```python
from build123d import *

# Parameters (mm, degrees)
SKETCH1_W           = 60
SKETCH1_H           = 400
BOSS_EXTRUDE1_DEPTH = 5
SKETCH2_R           = 30
BOSS_EXTRUDE2_DEPTH = 3
SKETCH3_R           = 3
BOSS_EXTRUDE3_DEPTH = 13
SKETCH4_R           = 4
BOSS_EXTRUDE4_DEPTH = 5
LPATTERN1_COUNT     = 8
LPATTERN1_PITCH     = 40


with BuildPart() as part:
    # Sketch1 → Boss-Extrude1 (new body)
    with BuildSketch(Plane.XY):
        Rectangle(SKETCH1_W, SKETCH1_H)
    extrude(amount=BOSS_EXTRUDE1_DEPTH)

    # Sketch2 → Boss-Extrude2 (add)
    with BuildSketch(Plane(origin=(0, 0, 0), x_dir=(-1, 0, 0), z_dir=(0, 0, -1))):
        with Locations((0, -110)):
            Circle(SKETCH2_R)
    extrude(amount=BOSS_EXTRUDE2_DEPTH)

    # Sketch3 → Boss-Extrude3 (add)
    with BuildSketch(Plane.XY.offset(5)):
        with Locations(Location((0, 165, 0), (0, 0, 180))):
            Circle(SKETCH3_R)
    boss_extrude3 = extrude(amount=BOSS_EXTRUDE3_DEPTH)

    # Sketch4 → Boss-Extrude4 (add)
    with BuildSketch(Plane.XY.offset(5)):
        with Locations(Location((0, 165, 0), (0, 0, 180))):
            Circle(SKETCH4_R)
    boss_extrude4 = extrude(amount=BOSS_EXTRUDE4_DEPTH)

    # LPattern1: Boss-Extrude3, Boss-Extrude4 ×8
    with Locations(*[(0, -i * LPATTERN1_PITCH, 0) for i in range(1, LPATTERN1_COUNT)]):
        add(boss_extrude3)
        add(boss_extrude4)


solid = part.part
```
Work out the finished part from the listing and answer in its coordinate system (mm). Give positions to 0.01 mm unless a question says otherwise; leave off trailing zeros. Order: outer loops, then holes, each group sorted by start corner. A loop starts at its lowest first (then second) coordinate and runs counter-clockwise, first axis right, second up. Notation, with made-up numbers: M 30.5,52.5 L 71.5,52.5 A15 ccw 71.5,65.5 Z; hole C 7,68 d7. An arc over 180 degrees is marked long. Return JSON: item names as keys, results as strings.
1) Section A-A, the plane x = 24 is taken. Write down the section's boundary in (y, z), plus the area to 3 significant figures.
Resolved:
{"outline": "M -200,0 L -128,0 L -128,-3 L -92,-3 L -92,0 L 200,0 L 200,5 L -200,5 Z", "area": "2,110 mm^2"}
2) Straight lines are drawn through the part: line 1 along Z through (x, y) = (-9.5, 164); line 2 along Z through (x, y) = (-1, 44); line 3 along Y through (x, z) = (27, -1). For each, find the intervals that lie inside material, in ascending order. Write a range as [from, to].
Resolved:
{"line 1": "[0, 5]", "line 2": "[0, 18]", "line 3": "[-123.08, -96.92]"}
3) For a pull along Y with two mould halves and no side action, classify faces 1 (the flat face through (0, -110, -3)), 2 (the cylindrical face through (-2.15, 121.627, 7.465)) as +Y half, -Y half, draft (parallel to the pull), parting line (faces both ways), or undercut.
Resolved:
{"face 1": "draft", "face 2": "undercut"}
4) Each of these flat-tipped pins is pushed along its axis until it touches: pin 1 (12 mm diameter, centred on x = -7, y = 151.5, fed in from -Z); pin 2 (18 mm diameter, centred on x = 13.5, y = -56.5, fed in from +Z). Where does it stop, or does it pass through?
Resolved:
{"pin 1": "z = 0", "pin 2": "z = 5"}
5) Section B-B, the plane x = -8.5 is taken. Write down the section's boundary in (y, z).
Resolved:
{"outline": "M -200,0 L -138.77,0 L -138.77,-3 L -81.23,-3 L -81.23,0 L 200,0 L 200,5 L -200,5 Z"}
